Verification items for the finished model (mm, model axes). Face numbers are marked on the shaded views. A direction names the side the tool comes from. Give positions to 0.01 mm unless a question says otherwise; leave off trailing zeros. Order: outer loops, then holes, each group sorted by start corner. A loop starts at its lowest first (then second) coordinate and runs counter-clockwise, first axis right, second up. Notation, with made-up numbers: M 41,-9 L 59,-9 A11 ccw 59,1 Z; hole C 39.25,2 d3. An arc over 180 degrees is marked long. Answer as a JSON object with one key per item and string values.
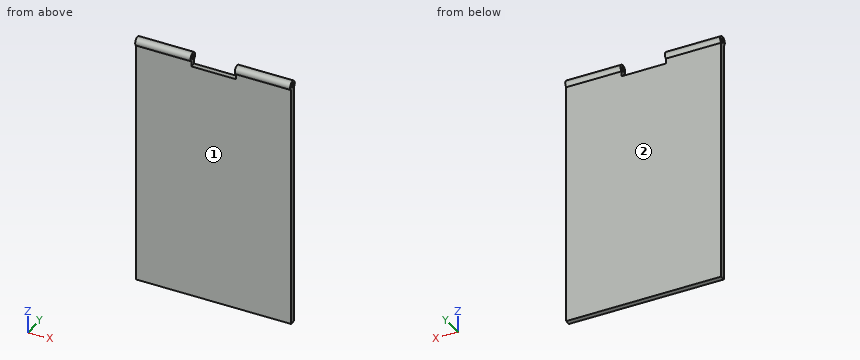
```python
from build123d import *

# Parameters (mm, degrees)
SKETCH1_W               = 88.9
SKETCH1_H               = 139.7
BOSS_EXTRUDE1_DEPTH     = 3
SKETCH3_R               = 1.27
BOSS_EXTRUDE2_DEPTH     = 88.9
CUT_EXTRUDE1_DEPTH      = 90.381450537
CUT_EXTRUDE1_DEPTH_BACK = 90.381450537
SKETCH4_W               = 25.4
SKETCH4_H               = 17.737449085


with BuildPart() as part:
    # Sketch1 → Boss-Extrude1 (new body)
    with BuildSketch(Plane(origin=(0, 0, 0), x_dir=(1, 0, 0), z_dir=(0, 1, 0))):
        Rectangle(SKETCH1_W, SKETCH1_H)
    extrude(amount=BOSS_EXTRUDE1_DEPTH)

    # Sketch3 → Boss-Extrude2 (add)
    with BuildSketch(Plane(origin=(44.45, 0, 0), x_dir=(0, 0, -1), z_dir=(1, 0, 0))):
        with BuildLine():
            Line((-69.85, 0), (-69.85, 3))
            Line((-69.85, 3), (-72.85, 3))
            ThreePointArc((-72.85, 3), (-77.439780476, 1.5), (-72.85, 0))
            Line((-72.85, 0), (-69.85, 0))
        make_face()
        with Locations((-74.899780476, 1.5)):
            Circle(SKETCH3_R, mode=Mode.SUBTRACT)
    extrude(amount=-BOSS_EXTRUDE2_DEPTH)

    # Sketch4 → Cut-Extrude1 (cut, two sides: drawn at the far end of the back side and taken through both)
    with BuildSketch(Plane(origin=(0, 0, 0), x_dir=(1, 0, 0), z_dir=(0, 1, 0)).offset(-CUT_EXTRUDE1_DEPTH_BACK)):
        with Locations((0, -78.718724543)):
            Rectangle(SKETCH4_W, SKETCH4_H)
    extrude(amount=CUT_EXTRUDE1_DEPTH + CUT_EXTRUDE1_DEPTH_BACK, mode=Mode.SUBTRACT)


solid = part.part
```
Q1. Section check A-A on y = 1.5. Record the cut outline in (x, z).
Resolved:
{"outline": "M -44.45,-69.85 L 44.45,-69.85 L 44.45,73.63 L 12.7,73.63 L 12.7,69.85 L -12.7,69.85 L -12.7,73.63 L -44.45,73.63 Z; M -44.45,76.17 L -12.7,76.17 L -12.7,77.44 L -44.45,77.44 Z; M 12.7,76.17 L 44.45,76.17 L 44.45,77.44 L 12.7,77.44 Z"}
Q2. Material ranges on L1, parallel to Z at x = 30, y = 1.7; L2, parallel to Y at x = -14, z = 46; L3, parallel to Z at x = -30.5, y = 0.75, recorded low to high.
Resolved:
{"L1": "z = -69.85 to 73.65, 76.15 to 77.43", "L2": "y = 0 to 3", "L3": "z = -69.85 to 73.87, 75.92 to 77.33"}
Q3. Section check C-C on x = 3.5. Record the cut outline in (y, z), then the cut area to 3 significant figures.
Resolved:
{"outline": "M 0,-69.85 L 3,-69.85 L 3,69.85 L 0,69.85 Z", "area": "419 mm²"}
Q4. Tool access check on the marked faces 1 and 2. Record the directions out of +Z, -Z, +X, -X, +Y, -Y that give a thin tool (end or side, any length) a straight path to the whole face; none if there is none.
Resolved:
{"face 1": "-Z, +X, -X, -Y", "face 2": "-Z, +X, -X, +Y"}
Q5. Section check B-B on x = 27.5. Record the cut outline in (y, z).
Resolved:
{"outline": "M 0,-69.85 L 3,-69.85 L 3,72.85 A2.54 ccw long 0,72.85 Z; hole C 1.5,74.9 d2.54"}
Q6. Gauge pin test, flat ends, axial feed: pin 1 Ø5 at (x, z) = (-35, 33) entering from +Y; pin 2 Ø5 at (x, z) = (17, 59) entering from -Y. Record the tip position at first contact, or that the pin passes through.
Resolved:
{"pin 1": "stops at y = 3", "pin 2": "stops at y = 0"}
Q7. Section check D-D on z = 40. Record the cut outline in (x, y).
Resolved:
{"outline": "M -44.45,0 L 44.45,0 L 44.45,3 L -44.45,3 Z"}
